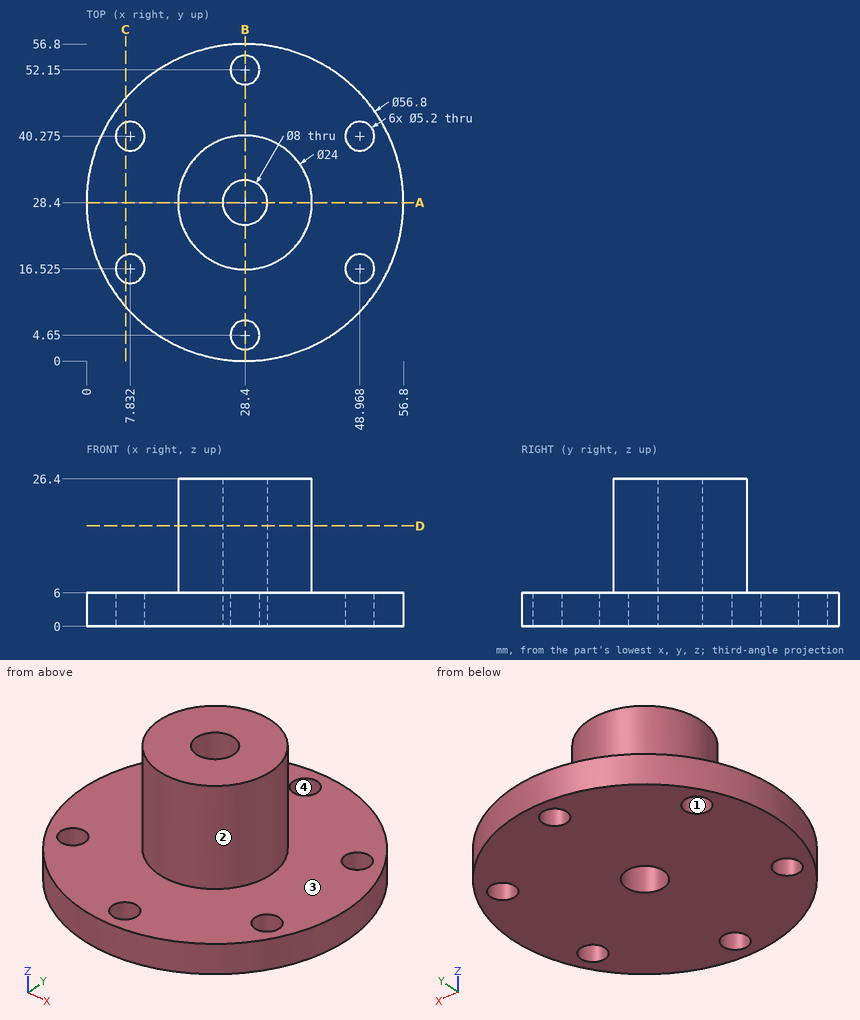
Can you work these out from the drawing? Everything is in mm from the part's minimum corner. Coordinates: 2 decimals unless noted, no trailing zeros. Write each loop counter-clockwise with the first axis right and the second up, starting at its lowest first coordinate (ties: lowest second). Pieces come first, ordered by that corner, then holes. Notation, with made-up numbers: (-17.5, 19) - (25.5, 19) arc R22 ccw to (25.5, 42) - close; hole circle Ø3 at (-19, 66). An arc over 180 degrees is marked (long way). One line per item, written item: value.
1) Suppose I cut it at D-D on z = 18. Write out the boundary of the cut face in (x, y), and give its area (3 significant figures).
Model answer:
outline: circle Ø24 at (28.4, 28.4); hole circle Ø8 at (28.4, 28.4)
area: 402 mm²
2) Suppose I cut it at B-B on x = 28.4. Write out the boundary of the cut face in (y, z), and give its area (3 significant figures).
Model answer:
outline: (0, 0) - (2.05, 0) - (2.05, 6) - (0, 6) - close; (7.25, 0) - (24.4, 0) - (24.4, 26.4) - (16.4, 26.4) - (16.4, 6) - (7.25, 6) - close; (32.4, 0) - (49.55, 0) - (49.55, 6) - (40.4, 6) - (40.4, 26.4) - (32.4, 26.4) - close; (54.75, 0) - (56.8, 0) - (56.8, 6) - (54.75, 6) - close
area: 557 mm²
3) Suppose I cut it at C-C on x = 7. Write out the boundary of the cut face in (y, z), and give its area (3 significant figures).
Model answer:
outline: (9.73, 0) - (14.06, 0) - (14.06, 6) - (9.73, 6) - close; (18.99, 0) - (37.81, 0) - (37.81, 6) - (18.99, 6) - close; (42.74, 0) - (47.07, 0) - (47.07, 6) - (42.74, 6) - close
area: 165 mm²
4) I'm going to push flat-ended pins straight in: P1, Ø4, axis at x = 38, z = 12.5, coming from the -Y side; P2, Ø5, axis at x = 42, z = 4, coming from the +Y side; P3, Ø1.5, axis at y = 31.5, z = 4.5, coming from the +X side. Where does each tip first touch, or does it pass through?
Model answer:
P1: stops at y = 19.11
P2: stops at y = 54.54
P3: stops at x = 56.7
5) We'd pull the mould along X, two halves only. Please class the marked faces 1, 2, 3 and 4: pulls with the +X half, pulls with the -X half, needs draft (parallel to the pull), parting line crosses it, or undercut.
Model answer:
face 1: undercut
face 2: parting line crosses it
face 3: needs draft
face 4: undercut
6) I need wall thicknesses on line 1 along Y through (x, z) = (28.4, 2.6); line 2 along Y through (x, z) = (28.4, 17.75); line 3 along Z through (x, y) = (16, 43). Which ranges of each line are inside material? Lowest first, please.
Model answer:
line 1: y = 0 to 2.05, 7.25 to 24.4, 32.4 to 49.55, 54.75 to 56.8
line 2: y = 16.4 to 24.4, 32.4 to 40.4
line 3: z = 0 to 6
7) Suppose I cut it at A-A on y = 28.4. Write out the boundary of the cut face in (x, z), and give its area (3 significant figures).
Model answer:
outline: (0, 0) - (24.4, 0) - (24.4, 26.4) - (16.4, 26.4) - (16.4, 6) - (0, 6) - close; (32.4, 0) - (56.8, 0) - (56.8, 6) - (40.4, 6) - (40.4, 26.4) - (32.4, 26.4) - close
area: 619 mm²
